Check sheet for the drawn part. Datum: minimum x, y, z corner. Units: mm. A direction names the side the tool comes from. Give positions to 0.01 mm unless a question says otherwise; leave off trailing zeros. Write each loop counter-clockwise with the first axis right and the second up, starting at its lowest first coordinate (ties: lowest second). Pieces come first, ordered by that corner, then holes. Notation, with made-up numbers: M 40,8.5 L 75,8.5 A30 cw 75,32.5 Z; hole C 74,14.25 d9. An arc over 180 degrees is marked long. Write item = value, one per line. Start each with the question number.
1) Gauge pin test, flat ends, axial feed: pin 1 (2.5 mm diameter, centred on x = 16.5, y = 15.5, fed in from +Z) (3 decimals); pin 2 (14 mm diameter, centred on x = 22, y = 34, fed in from +Z); pin 3 (4 mm diameter, centred on x = 19.05, z = 20.11, fed in from +Y) (1 decimal); pin 4 (1 mm diameter, centred on x = 12.5, z = 18.5, fed in from +Y). Record the tip position at first contact, or that the pin passes through.
2) Scan lines: L1, parallel to Y at x = 19.05, z = 2.8; L2, parallel to Z at x = 19.05, y = 1.6; L3, parallel to Z at x = 34, y = 9.5. Record each from-to range of solid material in increasing order.
3) Draft check along X on the marked faces 1, 2, 3 and 4. Enter one of: pulls with the +X half, pulls with the -X half, needs draft (parallel to the pull), parting line crosses it, or undercut.
4) Sectioned sample at D-D, the plane x = 30. Record the cut outline in (y, z).
5) Set-up check for the marked faces 5 and 6: record each of +Z, -Z, +X, -X, +Y, -Y from which the full face is reachable in a straight line by a thin tool's end or side.
6) Sectioned sample at C-C, the plane y = 13. Record the cut outline in (x, z).
7) Sectioned sample at A-A, the plane x = 19.05. Record the cut outline in (y, z).
8) Sectioned sample at B-B, the plane x = 23. Record the cut outline in (y, z).
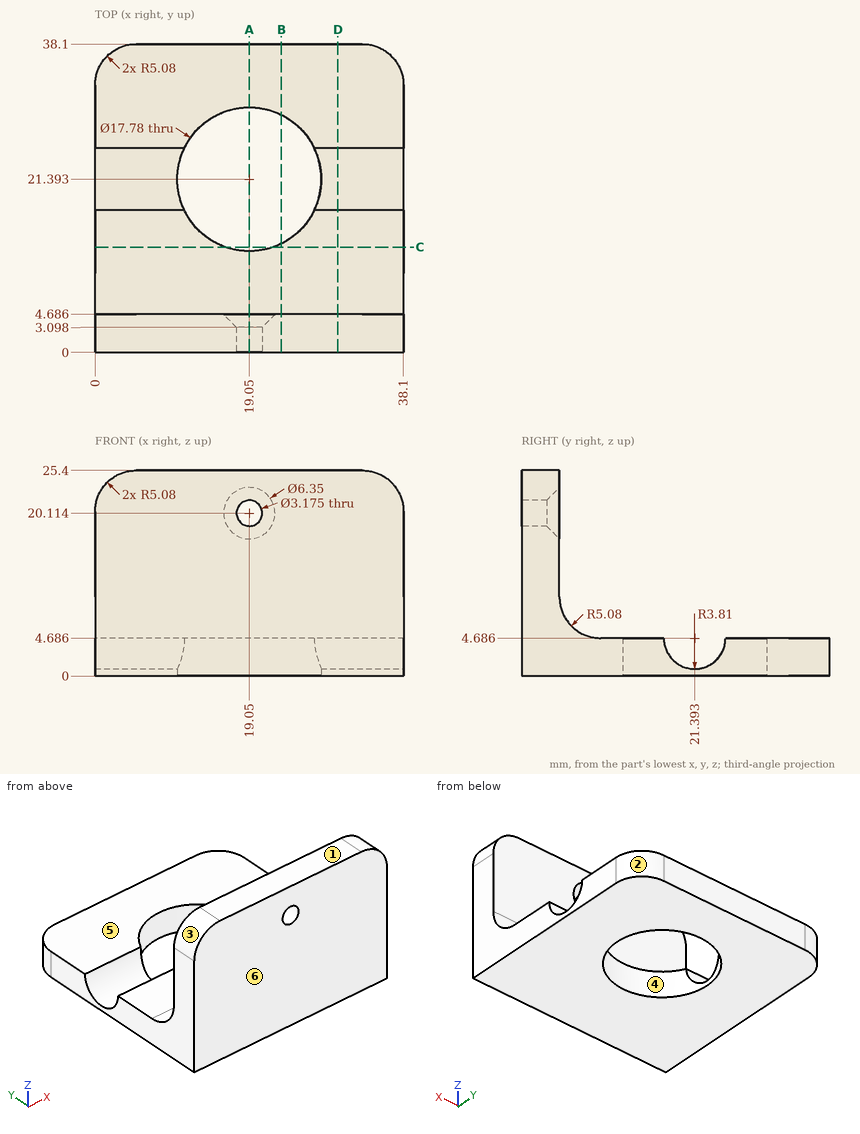
Data:
q1.pin_1 = through
q1.pin_2 = 4.69
q1.pin_3 = 3.5
q1.pin_4 = 4.69
q2.L1 = 0 to 12.5, 30.28 to 38.1
q2.L2 = 0 to 18.53, 21.7 to 25.4
q2.L3 = 0 to 4.69
q3.face_1 = needs draft
q3.face_2 = pulls with the +X half
q3.face_3 = pulls with the -X half
q3.face_4 = undercut
q4.outline = M 0,0 L 38.1,0 L 38.1,4.69 L 25.2,4.69 A3.81 cw 17.58,4.69 L 9.77,4.69 A5.08 cw 4.69,9.77 L 4.69,25.4 L 0,25.4 Z
q5.face_5 = +Z, +X, -X, +Y
q5.face_6 = +Z, -Z, +X, -X, -Y
q6.outline = M 0,0 L 16.12,0 L 16.12,4.69 L 0,4.69 Z; M 21.98,0 L 38.1,0 L 38.1,4.69 L 21.98,4.69 Z
q7.outline = M 0,0 L 12.5,0 L 12.5,4.69 L 9.77,4.69 A5.08 cw 4.69,9.77 L 4.69,16.94 L 3.1,18.53 L 0,18.53 Z; M 0,21.7 L 3.1,21.7 L 4.69,23.29 L 4.69,25.4 L 0,25.4 Z; M 30.28,0 L 38.1,0 L 38.1,4.69 L 30.28,4.69 Z
q8.outline = M 0,0 L 13.43,0 L 13.43,4.69 L 9.77,4.69 A5.08 cw 4.69,9.77 L 4.69,25.4 L 0,25.4 Z; M 29.36,0 L 38.1,0 L 38.1,4.69 L 29.36,4.69 Z
